Geometry check sheet. Reference: the model listing, model coordinates, mm. A direction names the side the tool comes from. Coordinates: 2 decimals unless noted, no trailing zeros. Loops run counter-clockwise (first coordinate to the right, second up) from the corner with the lowest first, then second, coordinate; pieces in that order, holes last. Notation, with made-up numbers: (42.25, -39) -> (51.25, -39) arc R10 ccw to (51.25, -22) -> close; hole circle Ø11 at (15.25, -28.5). An arc over 180 degrees is marked (long way). Answer as a JSON object with one key per item and string values.
Autodesk Inventor part; units mm, degrees
ref_plane "Work Plane1" through (0, 0, 15.5) normal (0, 0, 1) x (1, 0, 0)
ref_plane "YZ Plane" through (0, 0, 0) normal (1, 0, 0) x (0, 1, 0)
ref_plane "XZ Plane" through (0, 0, 0) normal (0, 1, 0) x (-1, 0, 0)
sketch "Sketch1" plane through (0, 0, 0) normal (0, 0, 1) x (1, 0, 0)
  line L0 (20.06, -29.05) -> (-20.06, -29.05)
  line L1 (-20.06, -29.05) -> (-20.06, 29.05)
  line L2 (-20.06, 29.05) -> (20.06, 29.05)
  line L3 (20.06, 29.05) -> (20.06, -29.05)
  line L4 (20.06, -29.05) -> (-20.06, 29.05) construction
  line L5 (-20.06, -29.05) -> (20.06, 29.05) construction
  point P0 (0, 0)
  dimension "d0" = 40.12
  dimension "d1" = 58.1
extrude "Extrusion1" add sketch "Sketch1" along normal blind 31
sketch "Sketch2" plane through (0, 0, 31) normal (0, 0, 1) x (1, 0, 0)
  line L0 (0, 0) -> (0, 8.85) construction
  circle A0 centre (0, 8.85) radius 9.4
  line L1 (-20.06, -29.05) -> (20.06, -29.05)
  dimension "d4" = 18.8
  dimension "d5" = 37.9
extrude "Extrusion2" add sketch "Sketch2" along normal blind 1.5
sketch "Sketch3" plane through (0, 8.85, 32.5) normal (0, 0, 1) x (1, 0, 0)
  circle A0 centre (0, 0) radius 9.4
  circle A1 centre (0, 0) radius 4
  point P0 (0, -8.85)
  dimension "d8" = 8
extrude "Extrusion3" add sketch "Sketch3" along normal blind 14.9 contours A1
sketch "Sketch4" plane through (0, 8.85, 47.4) normal (0, 0, 1) x (1, 0, 0)
  circle A0 centre (0, 0) radius 4 construction
  arc A1 (2.6458, 3) -> (-2.6458, 3) centre (0, 0) ccw
  line L0 (-2.6458, 3) -> (2.6458, 3)
  point P0 (0, -8.85)
  dimension "d11" = 7
extrude "Extrusion4" cut sketch "Sketch4" against normal blind 12
sketch "Sketch5" plane through (0, 0, 31) normal (0, 0, 1) x (1, 0, 0)
  circle A0 centre (0, 8.85) radius 9.4 construction
  line L0 (-20.06, -29.05) -> (20.06, -29.05) construction
  line L1 (20.06, -29.05) -> (20.06, 29.05) construction
  line L2 (20.06, 29.05) -> (-20.06, 29.05) construction
  line L3 (-20.06, 29.05) -> (-20.06, -29.05) construction
  line L4 (0, 29.05) -> (0, -29.05) construction
  line L5 (-20.06, -29.05) -> (20.06, -29.05) construction
  line L6 (14, -20) -> (-14, -20) construction
  line L7 (-14, -20) -> (-14, 20) construction
  line L8 (-14, 20) -> (14, 20) construction
  line L9 (14, 20) -> (14, -20) construction
  line L10 (14, -20) -> (-14, 20) construction
  line L11 (-14, -20) -> (14, 20) construction
  circle A1 centre (-14, 20) radius 2
  circle A2 centre (14, 20) radius 2
  circle A3 centre (14, -20) radius 2
  circle A4 centre (-14, -20) radius 2
  point P0 (0, 0)
  dimension "d14" = 28
  dimension "d15" = 40
  dimension "d16" = 4
extrude "Extrusion5" cut sketch "Sketch5" against normal blind 6
ref_plane "Work Plane1" through (0, 0, 15.5) normal (0, 0, 1) x (1, 0, 0)
mirror "Mirror1" about plane through (0, 0, 15.5) normal (0, 0, 1) of "Extrusion5", "Extrusion2"
sketch "Sketch6" plane through (-20.06, -29.05, 0) normal (0, -1, 0) x (1, 0, 0)
  line L0 (20.06, 0) -> (20.06, 11.3) construction
  circle A0 centre (20.06, 11.3) radius 15.5
  line L1 (40.12, 0) -> (0, 0)
  point P0 (20.06, -4.2)
  dimension "d19" = 31
  dimension "d20" = 4.2
extrude "Extrusion6" add sketch "Sketch6" along normal blind 57.2
properties part number "motor"
1. Section check D-D, the plane z = 11.3. Record the boundary of the cut face in (x, y), then the cut area to 3 significant figures.
Evaluation:
{"outline": "(-20.06, -29.05) -> (-15.5, -29.05) -> (-15.5, -86.25) -> (15.5, -86.25) -> (15.5, -29.05) -> (20.06, -29.05) -> (20.06, 29.05) -> (-20.06, 29.05) -> close", "area": "4,100 mm^2"}
2. Tool access check on faces 4 (the face through (-14, 22, 28)), 5 (the face through (-2.018, -57.25, -4.068)), 6 (the face through (14, 20, 6)). Record the directions out of +Z, -Z, +X, -X, +Y, -Y that give a thin tool (end or side, any length) a straight path to the whole face; none if there is none.
Evaluation:
{"face 4": "+Z", "face 5": "-Y", "face 6": "-Z"}
3. Thickness scan on probe 1 along Y at (x, z) = (-14, 3); probe 2 along Z at (x, y) = (0, -16); probe 3 along Y at (x, z) = (-17, 17). Record the ranges inside material, lowest first. Write a range as from..to.
Evaluation:
{"probe 1": "y = -29.05..-22, -18..18, 22..29.05", "probe 2": "z = 0..31", "probe 3": "y = -29.05..29.05"}
4. Section check A-A, the plane z = 2. Record the boundary of the cut face in (x, y).
Evaluation:
{"outline": "(-20.06, -29.05) -> (-12.4, -29.05) -> (-12.4, -86.25) -> (12.4, -86.25) -> (12.4, -29.05) -> (20.06, -29.05) -> (20.06, 29.05) -> (-20.06, 29.05) -> close; hole circle Ø4 at (-14, -20); hole circle Ø4 at (-14, 20); hole circle Ø4 at (14, -20); hole circle Ø4 at (14, 20)"}
5. Section check C-C, the plane x = 0. Record the boundary of the cut face in (y, z).
Evaluation:
{"outline": "(-86.25, -4.2) -> (-29.05, -4.2) -> (-29.05, 0) -> (-0.55, 0) -> (-0.55, -1.5) -> (18.25, -1.5) -> (18.25, 0) -> (29.05, 0) -> (29.05, 31) -> (18.25, 31) -> (18.25, 32.5) -> (12.85, 32.5) -> (12.85, 35.4) -> (11.85, 35.4) -> (11.85, 47.4) -> (4.85, 47.4) -> (4.85, 32.5) -> (-0.55, 32.5) -> (-0.55, 31) -> (-29.05, 31) -> (-29.05, 26.8) -> (-86.25, 26.8) -> close"}
6. Section check B-B, the plane y = 20. Record the boundary of the cut face in (x, z), then the cut area to 3 significant figures.
Evaluation:
{"outline": "(-20.06, 0) -> (-16, 0) -> (-16, 6) -> (-12, 6) -> (-12, 0) -> (12, 0) -> (12, 6) -> (16, 6) -> (16, 0) -> (20.06, 0) -> (20.06, 31) -> (16, 31) -> (16, 25) -> (12, 25) -> (12, 31) -> (-12, 31) -> (-12, 25) -> (-16, 25) -> (-16, 31) -> (-20.06, 31) -> close", "area": "1,150 mm^2"}
7. Depth check by flat-ended pin: P1, Ø4.5, axis at x = -1.5, z = -1.5, coming from the +Y side; P2, Ø2, axis at x = -13.5, y = 20.5, coming from the +Z side; P3, Ø6.5, axis at x = 14, y = 20, coming from the -Z side; P4, Ø3.5, axis at x = 14, y = -20, coming from the -Z side. Enter the tip coordinate at first touch or a pass-through.
Evaluation:
{"P1": "stops at y = 29.05", "P2": "stops at z = 25", "P3": "stops at z = 0", "P4": "stops at z = 6"}
8. Mould release check, pull along Y, two halves, no side actions. Record for faces 1 (the face through (0, 9, -1.5)), 2 (the face through (0, -29.05, 29)), 3 (the face through (14, -20, 6)): released by +Y, released by -Y, zero draft, split by the parting line, or undercut.
Evaluation:
{"face 1": "zero draft", "face 2": "released by -Y", "face 3": "undercut"}
